Answer from the drawing. Dimensions are ordinates in mm from the lowest x, y and z of the part. Give positions to 0.01 mm unless a question says otherwise; leave off trailing zeros. Order: outer loops, then holes, each group sorted by start corner. A loop starts at its lowest first (then second) coordinate and runs counter-clockwise, first axis right, second up.
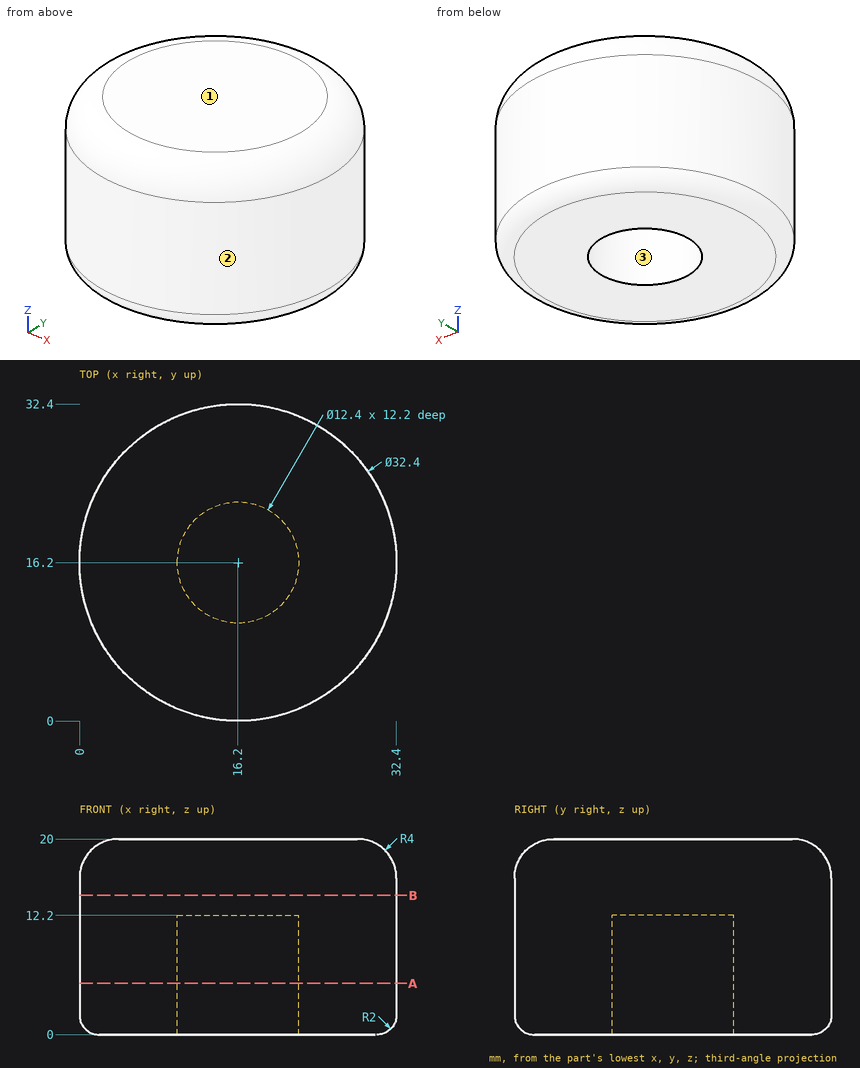
1) The part is cut by section A-A on z = 5.25. Determine the outline of the cut face in (x, y), and give its area (3 significant figures).
Final values:
outline: circle Ø32.4 at (16.2, 16.2); hole circle Ø12.4 at (16.2, 16.2)
area: 704 mm2
2) Consider L1, parallel to Y at x = 16.2, z = 3.5; L2, parallel to X at y = 21, z = 5; L3, parallel to X at y = 13.5, z = 12. Determine where each line is inside the solid, lowest interval first.
Final values:
L1: y = 0 to 10, 22.4 to 32.4
L2: x = 0.73 to 12.28, 20.12 to 31.67
L3: x = 0.23 to 10.62, 21.78 to 32.17
3) The part is cut by section B-B on z = 14.25. Determine the outline of the cut face in (x, y).
Final values:
outline: circle Ø32.4 at (16.2, 16.2)
4) Given pin 1 (1.5 mm diameter, centred on x = 12.5, z = 12, fed in from +Y); pin 2 (2 mm diameter, centred on y = 18, z = 16, fed in from +X); pin 3 (4 mm diameter, centred on x = 5.5, z = 6.5, fed in from -Y); pin 4 (5 mm diameter, centred on y = 17, z = 3, fed in from -X), each flat-ended and moving along its own axis, determine where each tip first touches the part or whether it passes through.
Final values:
pin 1: stops at y = 32.13
pin 2: stops at x = 32.38
pin 3: stops at y = 2.53
pin 4: stops at x = 0
5) For a pull along X with two mould halves and no side action, classify the marked faces 1, 2 and 3 as released by +X, released by -X, zero draft, split by the parting line, or undercut.
Final values:
face 1: zero draft
face 2: split by the parting line
face 3: undercut
